from build123d import *

# Parameters (mm, degrees)
SKETCH2_W           = 36
SKETCH2_H           = 5.5
SKETCH2_R           = 1.5
BOSS_EXTRUDE1_DEPTH = 4
SKETCH3_R           = 1.4
CUT_EXTRUDE1_DEPTH  = 5.5
FILLET1_R           = 2
FILLET2_R           = 0.5


with BuildPart() as part:
    # Sketch2 → Boss-Extrude1 (new body)
    with BuildSketch(Plane(origin=(0, 0, 0), x_dir=(1, 0, 0), z_dir=(0, 1, 0))):
        Rectangle(SKETCH2_W, SKETCH2_H)
        with Locations((-15.25, 0)):
            Circle(SKETCH2_R, mode=Mode.SUBTRACT)
        with Locations((15.25, 0)):
            Circle(SKETCH2_R, mode=Mode.SUBTRACT)
    extrude(amount=BOSS_EXTRUDE1_DEPTH)

    # Sketch3 → Cut-Extrude1 (cut)
    with BuildSketch(Plane.XY.offset(2.75)):
        with Locations((-5, 1.4)):
            Circle(SKETCH3_R)
        with BuildLine():
            ThreePointArc((-5.000000005, 0), (-5.989949495, 0.410050508), (-6.4, 1.4))
            Line((-6.4, 1.4), (-6.4, 0))
            Line((-6.4, 0), (-5.000000005, 0))
        make_face()
        with BuildLine():
            Line((-3.6, 0), (-3.6, 1.4))
            ThreePointArc((-3.6, 1.4), (-4.010050508, 0.410050505), (-5.000000005, 0))
            Line((-5.000000005, 0), (-3.6, 0))
        make_face()
        with BuildLine():
            Line((-1.5, 2.8), (-5, 2.8))
            ThreePointArc((-5, 2.8), (-4.010050506, 2.389949494), (-3.6, 1.4))
            Line((-3.6, 1.4), (-3.6, 0))
            Line((-3.6, 0), (-2.9, 0))
            Line((-2.9, 0), (-2.9, 1.4))
            ThreePointArc((-2.9, 1.4), (-2.489949494, 2.389949494), (-1.5, 2.8))
        make_face()
        with BuildLine():
            ThreePointArc((-1.500000004, 0), (-2.489949495, 0.410050508), (-2.9, 1.4))
            Line((-2.9, 1.4), (-2.9, 0))
            Line((-2.9, 0), (-1.500000004, 0))
        make_face()
        with Locations((-1.5, 1.4)):
            Circle(SKETCH3_R)
        with BuildLine():
            Line((-0.1, 0), (-0.1, 1.4))
            ThreePointArc((-0.1, 1.4), (-0.510050508, 0.410050505), (-1.500000004, 0))
            Line((-1.500000004, 0), (-0.1, 0))
        make_face()
    extrude(amount=-CUT_EXTRUDE1_DEPTH, mode=Mode.SUBTRACT)

    # Fillet1
    fillet1_edges = [part.edges().sort_by_distance(p)[0] for p in [
        (18, 2, 2.75),
        (-18, 2, 2.75),
        (-18, 2, -2.75),
        (18, 2, -2.75),
    ]]
    fillet(fillet1_edges, radius=FILLET1_R)

    # Fillet2
    fillet2_edges = [part.edges().sort_by_distance(p)[0] for p in [
        (0, 4, -2.75),
        (18, 4, 0),
        (-18, 4, 0),
        (0, 4, 2.75),
        (-17.414213562, 4, 2.164213562),
        (-17.414213562, 4, -2.164213562),
        (17.414213562, 4, 2.164213562),
        (17.414213562, 4, -2.164213562),
    ]]
    fillet(fillet2_edges, radius=FILLET2_R)


solid = part.part
Source: CAD feature listing. Evaluate the final solid. Frame: model axes, mm. A direction names the side the tool comes from. Coordinates: 2 decimals unless noted, no trailing zeros. Loops run counter-clockwise (first coordinate to the right, second up) from the corner with the lowest first, then second, coordinate; pieces in that order, holes last. Notation, with made-up numbers: (89.25, -36.75) - (102.25, -36.75) arc R12 ccw to (102.25, -25.75) - close; hole circle Ø5 at (57.25, 19.25). An arc over 180 degrees is marked (long way). Return JSON: item names as keys, results as strings.
Q1. Section C-C, the plane y = 1.85. Return loops of the section in (x, z), plus the area to 3 significant figures.
Results:
{"outline": "(-18, -0.75) arc R2 ccw to (-16, -2.75) - (-6.33, -2.75) - (-6.33, 2.75) - (-16, 2.75) arc R2 ccw to (-18, 0.75) - close; (-0.17, -2.75) - (16, -2.75) arc R2 ccw to (18, -0.75) - (18, 0.75) arc R2 ccw to (16, 2.75) - (-0.17, 2.75) - close; hole circle Ø3 at (-15.25, 0); hole circle Ø3 at (15.25, 0)", "area": "147 mm2"}
Q2. Access query for faces 1 (the flat face through (18, 2, 0)), 2 (the cylindrical face through (-5.98, 2.4, 0.04)). Directions: +Z, -Z, +X, -X, +Y, -Y. A direction counts if a zero-diameter tool reaches every point of the face in a straight line with its end or side. Return the directions, or none.
Results:
{"face 1": "+Z, -Z, +X, +Y, -Y", "face 2": "+Z, -Z, -Y"}
Q3. Material intervals for line 1 along X through (y, z) = (3.15, 0.15); line 2 along X through (y, z) = (2.9, 1.05); line 3 along Z through (x, y) = (15.25, 1.3), sorted ascending.
Results:
{"line 1": "-18 to -16.74, -13.76 to 13.76, 16.74 to 18", "line 2": "-17.98 to -16.32, -14.18 to 14.18, 16.32 to 17.98", "line 3": "-2.75 to -1.5, 1.5 to 2.75"}
Q4. Section A-A, the plane z = 0. Return loops of the section in (x, y), plus the area to 3 significant figures.
Results:
{"outline": "(-18, 0) - (-16.75, 0) - (-16.75, 4) - (-17.5, 4) arc R0.5 ccw to (-18, 3.5) - close; (-13.75, 0) - (-6.4, 0) - (-6.4, 1.4) arc R1.4 cw to (-5, 2.8) - (-1.5, 2.8) arc R1.4 cw to (-0.1, 1.4) - (-0.1, 0) - (13.75, 0) - (13.75, 4) - (-13.75, 4) - close; (16.75, 0) - (18, 0) - (18, 3.5) arc R0.5 ccw to (17.5, 4) - (16.75, 4) - close", "area": "103 mm2"}
Q5. Contact query for flat-ended pins moving along their axis: P1, Ø1, axis at x = -3, z = -1, coming from the -Y side; P2, Ø1.8, axis at x = 15.25, z = 0, coming from the -Y side. Output: stop coordinate, or through.
Results:
{"P1": "y = 2.8", "P2": "through"}
Q6. Mould query, pull axis Z, two halves, no side actions, for faces 3 (the cylindrical face through (17.4, 1.77, -2.18)), 4 (the cylindrical face through (13.75, 1.97, -0.07)), 5 (the cylindrical face through (-0.5, 2.38, 0.04)). Classes: released by +Z, released by -Z, zero draft, split by the parting line, or undercut.
Results:
{"face 3": "released by -Z", "face 4": "undercut", "face 5": "zero draft"}
Q7. Section B-B, the plane x = -15.25. Return loops of the section in (y, z).
Results:
{"outline": "(0, -2.75) - (3.5, -2.75) arc R0.5 ccw to (4, -2.25) - (4, -1.5) - (0, -1.5) - close; (0, 1.5) - (4, 1.5) - (4, 2.25) arc R0.5 ccw to (3.5, 2.75) - (0, 2.75) - close"}
